The listing builds one solid part. Answer for the finished solid, in the listing's coordinates (mm). Face numbers are marked on the shaded views. A direction names the side the tool comes from. Give positions to 0.01 mm unless a question says otherwise; leave off trailing zeros. Write each loop counter-clockwise with the first axis right and the second up, starting at its lowest first coordinate (ties: lowest second). Pieces come first, ordered by that corner, then holes. Notation, with made-up numbers: (18, -10.5) - (59, -10.5) arc R10 cw to (59, -3.5) - close; hole circle Ø7 at (63, 30). An arc over 180 degrees is marked (long way). Use a Markdown table: item, result. Add a question column.
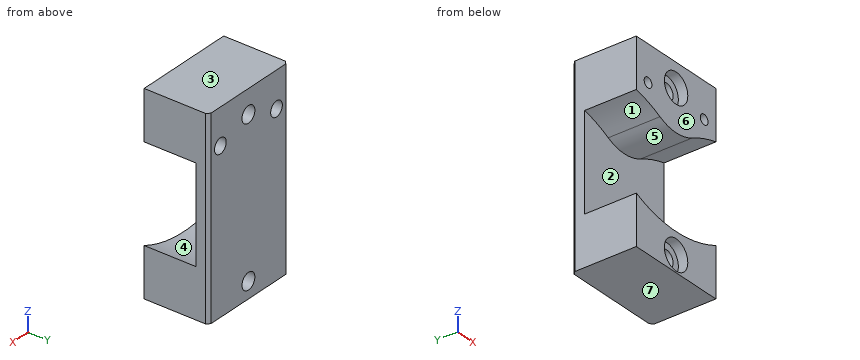
from build123d import *

# Parameters (mm, degrees)
SKIZZE1_R                                            = 52.5
SKIZZE1_R_2                                          = 17.5
AUFSATZ_LINEAR_AUSTRAGEN1_DEPTH                      = 65
SKIZZE18_W                                           = 35.5
SKIZZE18_H                                           = 65
SCHNITT_LINEAR_AUSTRAGEN11_DEPTH                     = 106
SKIZZE25_W                                           = 34
SKIZZE25_H                                           = 81
SCHNITT_LINEAR_AUSTRAGEN12_DEPTH                     = 66
F_5_0_5_DURCHMESSER_BOHRUNG1_D                       = 5
F_5_0_5_DURCHMESSER_BOHRUNG1_DEPTH                   = 12
F_5_0_5_DURCHMESSER_BOHRUNG1_TIP                     = 1.502151548
M4_GEWINDEBOHRUNG1_D                                 = 3.3
STIRNSENKUNG_F_R_M5_ZYLINDERSCHRAUBE_MIT_D           = 5.5
STIRNSENKUNG_F_R_M5_ZYLINDERSCHRAUBE_MIT_CBORE_D     = 10
STIRNSENKUNG_F_R_M5_ZYLINDERSCHRAUBE_MIT_CBORE_DEPTH = 6
FASE1_SIZE                                           = 1
CUT_EXTRUDE1_DEPTH                                   = 20.2
SKETCH1_W                                            = 34
SKETCH1_H                                            = 65
CUT_EXTRUDE2_DEPTH                                   = 2.82858


with BuildPart() as part:
    # Skizze1 → Aufsatz-Linear austragen1 (new body)
    with BuildSketch(Plane.XY):
        Circle(SKIZZE1_R)
        Circle(SKIZZE1_R_2, mode=Mode.SUBTRACT)
    extrude(amount=AUFSATZ_LINEAR_AUSTRAGEN1_DEPTH)

    # Skizze18 → Schnitt-Linear austragen11 (cut, through all)
    with BuildSketch(Plane(origin=(0, -52.5, 0), x_dir=(1, 0, 0), z_dir=(0, 1, 0))):
        with Locations((-34.75, -32.5)):
            Rectangle(SKIZZE18_W, SKIZZE18_H)
        with Locations((34.75, -32.5)):
            Rectangle(SKIZZE18_W, SKIZZE18_H)
    extrude(amount=SCHNITT_LINEAR_AUSTRAGEN11_DEPTH, mode=Mode.SUBTRACT)

    # Skizze25 → Schnitt-Linear austragen12 (cut, through all)
    with BuildSketch(Plane.XY):
        with Locations((0, 12.5)):
            Rectangle(SKIZZE25_W, SKIZZE25_H)
    extrude(amount=SCHNITT_LINEAR_AUSTRAGEN12_DEPTH, mode=Mode.SUBTRACT)

    # 5.0 _5_ Durchmesser Bohrung1
    with Locations(Plane(origin=(0, -28, 0), x_dir=(1, 0, 0), z_dir=(0, 1, 0))):
        with Locations((12, -53), (-12, -53)):
            Hole(F_5_0_5_DURCHMESSER_BOHRUNG1_D / 2, depth=F_5_0_5_DURCHMESSER_BOHRUNG1_DEPTH)
            with Locations((0, 0, -(F_5_0_5_DURCHMESSER_BOHRUNG1_DEPTH + F_5_0_5_DURCHMESSER_BOHRUNG1_TIP / 2))):  # 118° drill point
                Cone(0, F_5_0_5_DURCHMESSER_BOHRUNG1_D / 2, F_5_0_5_DURCHMESSER_BOHRUNG1_TIP, mode=Mode.SUBTRACT)

    # M4 Gewindebohrung1 (through all)
    with Locations(Plane.XZ.offset(52.5)):
        with Locations((-12, 53), (12, 53)):
            Hole(M4_GEWINDEBOHRUNG1_D / 2)

    # Stirnsenkung f_r M5 Zylinderschraube mit (through all)
    with Locations(Plane.XZ.offset(52.5)):
        with Locations((0, 5.5), (0, 57)):
            CounterBoreHole(STIRNSENKUNG_F_R_M5_ZYLINDERSCHRAUBE_MIT_D / 2, STIRNSENKUNG_F_R_M5_ZYLINDERSCHRAUBE_MIT_CBORE_D / 2, STIRNSENKUNG_F_R_M5_ZYLINDERSCHRAUBE_MIT_CBORE_DEPTH)

    # Fase1
    fase1_edges = [part.edges().sort_by_distance(p)[0] for p in [
        (-17, -28, 32.5),
        (17, -28, 32.5),
    ]]
    chamfer(fase1_edges, length=FASE1_SIZE)

    # Skizze3_2 → Cut-Extrude1 (cut)
    with BuildSketch(Plane(origin=(0, -52.5, 0), x_dir=(1, 0, 0), z_dir=(0, 1, 0))):
        with BuildLine():
            Line((17, -48.5), (17, -16.5))
            ThreePointArc((17, -16.5), (0, -12.70773398), (-17, -16.5))
            Line((-17, -16.5), (-17, -48.5))
            ThreePointArc((-17, -48.5), (-11.82232192, -47.038215467), (-6.887645327, -44.894823008))
            ThreePointArc((-6.887645327, -44.894823008), (0, -43.22), (6.887645327, -44.894823008))
            ThreePointArc((6.887645327, -44.894823008), (11.82232192, -47.038215467), (17, -48.5))
        make_face()
    extrude(amount=CUT_EXTRUDE1_DEPTH, mode=Mode.SUBTRACT)

    # Sketch1 → Cut-Extrude2 (cut)
    with BuildSketch(Plane(origin=(0, -52.5, 0), x_dir=(1, 0, 0), z_dir=(0, 1, 0))):
        with Locations((0, -32.5)):
            Rectangle(SKETCH1_W, SKETCH1_H)
    extrude(amount=CUT_EXTRUDE2_DEPTH, mode=Mode.SUBTRACT)


solid = part.part
1. The part is cut by section C-C (z = 57). Give the vertices of the cut face in (x, y).
2. The part is cut by section A-A (y = -35.75). Give the vertices of the cut face in (x, z).
3. Consider L1, parallel to X at y = -34.25, z = 53; L2, parallel to X at y = -42.5, z = 53; L3, parallel to Z at x = -12, y = -44.5. Determine where each line is inside the solid, lowest interval first. Write a range as [from, to].
4. For a pull along Z with two mould halves and no side action, classify the marked faces 4, 5, 6 and 7 as released by +Z, released by -Z, zero draft, split by the parting line, or undercut.
5. Which of the six approach directions +Z, -Z, +X, -X, +Y, -Y give full straight-line access (tool end or side, diameter ignored) to the marked faces 1, 2 and 3?
6. The part is cut by section D-D (y = -30.5). Give the vertices of the cut face in (x, z).
7. Given P1, Ø4.5, axis at x = -12, z = 53, coming from the +Y side; P2, Ø4, axis at x = -5, z = 31.5, coming from the -Y side; P3, Ø5, axis at x = -1, z = 4.5, coming from the -Y side, each flat-ended and moving along its own axis, determine where each tip first touches the part or whether it passes through.
8. The part is cut by section B-B (x = 0). Give the vertices of the cut face in (y, z).
Check values:
| question | item | result |
|---|---|---|
| 1 | outline | (-17, -49.67) - (-5, -49.67) - (-5, -46.5) - (-2.75, -46.5) - (-2.75, -28) - (-16, -28) - (-17, -29) - close; (2.75, -46.5) - (5, -46.5) - (5, -49.67) - (17, -49.67) - (17, -29) - (16, -28) - (2.75, -28) - close |
| 2 | outline | (-17, 0) - (17, 0) - (17, 16.5) arc R40 cw to (-17, 16.5) - close; (-17, 48.5) arc R40 cw to (-6.89, 44.89) arc R15 ccw to (6.89, 44.89) arc R40 cw to (17, 48.5) - (17, 65) - (-17, 65) - close; hole circle Ø5 at (-12, 53); hole circle Ø5.5 at (0, 5.5); hole circle Ø5.5 at (0, 57); hole circle Ø5 at (12, 53) |
| 3 | L1 | x = [-17, -14.5], [-9.5, 9.5], [14.5, 17] |
| 3 | L2 | x = [-17, -13.65], [-10.35, 10.35], [13.65, 17] |
| 3 | L3 | z = [0, 14.55], [47.1, 51.35], [54.65, 65] |
| 4 | face 4 | undercut |
| 4 | face 5 | undercut |
| 4 | face 6 | zero draft |
| 4 | face 7 | released by -Z |
| 5 | face 1 | -X, -Y |
| 5 | face 2 | -Y |
| 5 | face 3 | +Z, +X, -X, +Y, -Y |
| 6 | outline | (-17, 0) - (17, 0) - (17, 65) - (-17, 65) - close; hole circle Ø5 at (-12, 53); hole circle Ø5.5 at (0, 5.5); hole circle Ø5.5 at (0, 57); hole circle Ø5 at (12, 53) |
| 7 | P1 | stops at y = -40.15 |
| 7 | P2 | stops at y = -32.3 |
| 7 | P3 | stops at y = -46.5 |
| 8 | outline | (-49.67, 0) - (-28, 0) - (-28, 2.75) - (-46.5, 2.75) - (-46.5, 0.5) - (-49.67, 0.5) - close; (-49.67, 10.5) - (-46.5, 10.5) - (-46.5, 8.25) - (-28, 8.25) - (-28, 54.25) - (-46.5, 54.25) - (-46.5, 52) - (-49.67, 52) - (-49.67, 43.22) - (-32.3, 43.22) - (-32.3, 12.71) - (-49.67, 12.71) - close; (-49.67, 62) - (-46.5, 62) - (-46.5, 59.75) - (-28, 59.75) - (-28, 65) - (-49.67, 65) - close |
